For this review, take the finished solid that the model builds, in its own axes (mm). A direction names the side the tool comes from. Coordinates: 2 decimals unless noted, no trailing zeros. Loops run counter-clockwise (first coordinate to the right, second up) from the corner with the lowest first, then second, coordinate; pieces in that order, holes last. Notation, with made-up numbers: M 51.5,50.25 L 76.5,50.25 A29 ccw 76.5,78.25 Z; hole C -39.5,8 d1. An arc over 180 degrees is marked long. Answer as a JSON object with one key per item and string values. Group by question number.
Item 1: Mouldability with a two-part tool opening along Y and no side actions: class faces 3 (the face through (0, 22, 1)), 4 (the face through (20, -2.4, 30.8)), 5 (the face through (-20, 0, 50)), 6 (the face through (20, -2.4, -37.2)) as +Y half, -Y half, draft (parallel to the pull), parting line (faces both ways), or undercut.
Item 2: Tool access review of faces 1 (the face through (0, -22, 1)), 2 (the face through (18, 0, 1)): name each direction out of +Z, -Z, +X, -X, +Y, -Y from which nothing blocks a thin tool from reaching the whole face with its end or side.
Item 3: Wall thickness on L1, parallel to X at y = -7, z = 0; L2, parallel to Y at x = 19, z = -34: over which ranges is each line inside the solid? List them lowest first. Write a range as from..to.
Item 4: Add section D-D (y = 0). State the section outline as (x, z) points.
Item 5: Add section C-C (z = -34). State the section outline as (x, y) points, then the cut area to 3 significant figures.
Item 6: Add section A-A (y = -9.5). State the section outline as (x, z) points, then the cut area to 3 significant figures.
from build123d import *

# Parameters (mm, degrees)
SKETCH1_W           = 44
SKETCH1_H           = 44
SKETCH1_W_2         = 36
SKETCH1_H_2         = 36
EXTRUDE_THIN1_DEPTH = 50
SKETCH2_R           = 4
CUT_EXTRUDE1_DEPTH  = 45


with BuildPart() as part:
    # Sketch1 → Extrude-Thin1 (new body, symmetric)
    with BuildSketch(Plane.XY):
        Rectangle(SKETCH1_W, SKETCH1_H)
        Rectangle(SKETCH1_W_2, SKETCH1_H_2, mode=Mode.SUBTRACT)
    extrude(amount=EXTRUDE_THIN1_DEPTH, both=True)

    # Sketch2 → Cut-Extrude1 (cut, through all)
    with BuildSketch(Plane.ZY.offset(22)):
        with Locations((34, 0)):
            Circle(SKETCH2_R)
        with Locations((-34, 0)):
            Circle(SKETCH2_R)
    extrude(amount=-CUT_EXTRUDE1_DEPTH, mode=Mode.SUBTRACT)


solid = part.part
From the geometry:
{
 "1": {"face 3": "+Y half", "face 4": "undercut", "face 5": "draft", "face 6": "undercut"},
 "2": {"face 1": "+Z, -Z, +X, -X, -Y", "face 2": "+Z, -Z"},
 "3": {"L1": "x = -22..-18, 18..22", "L2": "y = -22..-4, 4..22"},
 "4": {"outline": "M -22,-50 L -18,-50 L -18,-38 L -22,-38 Z; M -22,-30 L -18,-30 L -18,30 L -22,30 Z; M -22,38 L -18,38 L -18,50 L -22,50 Z; M 18,-50 L 22,-50 L 22,-38 L 18,-38 Z; M 18,-30 L 22,-30 L 22,30 L 18,30 Z; M 18,38 L 22,38 L 22,50 L 18,50 Z"},
 "5": {"outline": "M -22,-22 L 22,-22 L 22,-4 L 18,-4 L 18,-18 L -18,-18 L -18,-4 L -22,-4 Z; M -22,4 L -18,4 L -18,18 L 18,18 L 18,4 L 22,4 L 22,22 L -22,22 Z", "area": "576 mm²"},
 "6": {"outline": "M -22,-50 L -18,-50 L -18,50 L -22,50 Z; M 18,-50 L 22,-50 L 22,50 L 18,50 Z", "area": "800 mm²"}
}
